Read the model definition and answer for the solid it produces. Units are mm, in the model's axes. A direction names the side the tool comes from. Coordinates: 2 decimals unless noted, no trailing zeros. Order: outer loops, then holes, each group sorted by start corner. A loop starts at its lowest first (then second) coordinate and runs counter-clockwise, first axis right, second up. Notation, with made-up numbers: (-19, 5) -> (-13, 5) arc R20 cw to (-13, 20) -> close; hole circle Ø11 at (-3.5, -16). An arc over 180 degrees is marked (long way). Answer as a JSON object with one key per item and string values. Group by question number.
1) A tool of negligible diameter and unlimited length cuts with its end or side. For faces 1 (the flat face through (10, 2.839, 11)), 2 (the flat face through (-8, 3.46, 10.99)), 3 (the flat face through (-10, 4.059, 11)), 4 (the flat face through (-13.02, 1.79, 10.99)), from which of +Z, -Z, +X, -X, +Y, -Y can it reach the whole face along a straight path? Write none if from no direction.
2) Determine the mould class of faces 5 (the cylindrical face through (-22.15, -6.99, 5.07)), 6 (the flat face through (-6, 1.547, 11)), 7 (the flat face through (-21, -0.534, 11)) for opening direction X: released by +X, released by -X, zero draft, split by the parting line, or undercut.
3) Consider L1, parallel to X at y = 2, z = 10.5; L2, parallel to X at y = 1.75, z = 10.5; L3, parallel to Z at x = 5, y = 5.75. Determine where each line is inside the solid, lowest interval first.
4) Section D-D on y = 5 is taken. Determine the outline of the cut face in (x, z).
5) Section C-C on x = -0.5 is taken. Determine the outline of the cut face in (y, z), and give its area (3 significant figures).
6) Given pin 1 (0.6 mm diameter, centred on x = -4, z = 11, fed in from +Y); pin 2 (6 mm diameter, centred on y = -7.5, z = 1.5, fed in from -X); pin 3 (0.6 mm diameter, centred on y = -2, z = 11, fed in from -X); pin 4 (1.9 mm diameter, centred on x = -15.5, z = 10.5, fed in from +Y), each flat-ended and moving along its own axis, determine where each tip first touches the part or whether it passes through.
7) Section B-B on y = 2 is taken. Determine the outline of the cut face in (x, z), and give its area (3 significant figures).
from build123d import *

# Parameters (mm, degrees)
ESQUISSE1_W             = 50
ESQUISSE1_H             = 20
BOSS_EXTRU_1_DEPTH      = 10
CONG_1_R                = 10
ESQUISSE2_R             = 4
ENL_V_MAT_EXTRU_1_DEPTH = 29.722813233
BOSS_EXTRU_2_DEPTH      = 2


with BuildPart() as part:
    # Esquisse1 → Boss.-Extru.1 (new body)
    with BuildSketch(Plane.XY):
        Rectangle(ESQUISSE1_W, ESQUISSE1_H)
    extrude(amount=BOSS_EXTRU_1_DEPTH)

    # Congé1
    cong_1_edges = [part.edges().sort_by_distance(p)[0] for p in [
        (-25, 10, 5),
        (25, 10, 5),
        (25, -10, 5),
        (-25, -10, 5),
    ]]
    fillet(cong_1_edges, radius=CONG_1_R - 0.0001)  # a hair under: the kernel refuses the full size

    # Esquisse2 → Enlèv. mat.-Extru.1 (cut, through all)
    with BuildSketch(Plane.XY.offset(10)):
        with Locations((18.655435278, 0)):
            Circle(ESQUISSE2_R)
    extrude(amount=-ENL_V_MAT_EXTRU_1_DEPTH, mode=Mode.SUBTRACT)

    # Esquisse3 → Boss.-Extru.2 (add)
    with BuildSketch(Plane.XY.offset(10)):
        Polygon((-23.137412504, -2.382112664), (-18.75901173, -2.382112664), (-13.477180662, 4.059144735), (-16.118096196, 4.059144735), (-19.884214818, -0.533682853), (-21.669171822, -0.533682853), align=None)
        Polygon((-18.126480253, -2.382112664), (-14.004075518, -2.382112664), (-8.774539808, 4.059144735), (-11.177021234, 4.059144735), (-14.905851553, -0.533682853), (-16.625774862, -0.533682853), align=None)
        Polygon((-12.458173742, -2.382112664), (-10.074908504, -2.382112664), (-8.200459195, 0), (-6.854279805, 0), (-5.173191017, -2.382112664), (-2.538637347, -2.382112664), (-4.219726135, 0), (-1.691447938, 0), (1.502633165, 4.059144735), (-7.5273695, 4.059144735), (-8.487196781, 2.839364232), (-1.691447938, 2.839364232), (-2.538637347, 1.547054349), (-9.36637019, 1.547054349), align=None)
        Polygon((3.258494312, 4.059144735), (3.967032626, 4.059144735), (-1.250385868, -2.382112664), (-1.958924181, -2.382112664), align=None)
        Polygon((7.831787065, -2.382112664), (0.681991352, -2.382112664), (0.681991352, -1.609161776), (5.512934401, 4.059144735), (12.533904966, 4.059144735), (12.018604374, 2.839364232), (6.944143524, 2.839364232), (4.069387486, -0.533682853), (9.023419684, -0.533682853), align=None)
    extrude(amount=BOSS_EXTRU_2_DEPTH)


solid = part.part
Worked answers:
{
 "1": {"face 1": "+Z, +X", "face 2": "+Z, +Y", "face 3": "+Z, +X, -X, +Y", "face 4": "+Z"},
 "2": {"face 5": "released by -X", "face 6": "undercut", "face 7": "zero draft"},
 "3": {"L1": "x = -17.81 to -15.17, -12.85 to -10.45, -2.24 to -0.12, 1.59 to 2.3, 3.76 to 6.23", "L2": "x = -18.01 to -15.37, -13.05 to -10.65, -2.41 to -0.31, 1.39 to 2.1, 3.54 to 6.02", "L3": "z = 0 to 10"},
 "4": {"outline": "(-23.66, 0) -> (23.66, 0) -> (23.66, 10) -> (-23.66, 10) -> close"},
 "5": {"outline": "(-10, 0) -> (10, 0) -> (10, 10) -> (4.06, 10) -> (4.06, 12) -> (1.51, 12) -> (1.51, 10) -> (-0.58, 10) -> (-0.58, 12) -> (-1.46, 12) -> (-1.46, 10) -> (-10, 10) -> close", "area": "207 mm²"},
 "6": {"pin 1": "stops at y = 4.06", "pin 2": "stops at x = -23.93", "pin 3": "stops at x = -23.07", "pin 4": "stops at y = 10"},
 "7": {"outline": "(-24.8, 0) -> (15.19, 0) -> (15.19, 10) -> (6.23, 10) -> (6.23, 12) -> (3.76, 12) -> (3.76, 10) -> (2.3, 10) -> (2.3, 12) -> (1.59, 12) -> (1.59, 10) -> (-0.12, 10) -> (-0.12, 12) -> (-2.24, 12) -> (-2.24, 10) -> (-10.45, 10) -> (-10.45, 12) -> (-12.85, 12) -> (-12.85, 10) -> (-15.17, 10) -> (-15.17, 12) -> (-17.81, 12) -> (-17.81, 10) -> (-24.8, 10) -> close; (22.12, 0) -> (24.8, 0) -> (24.8, 10) -> (22.12, 10) -> close", "area": "447 mm²"}
}
